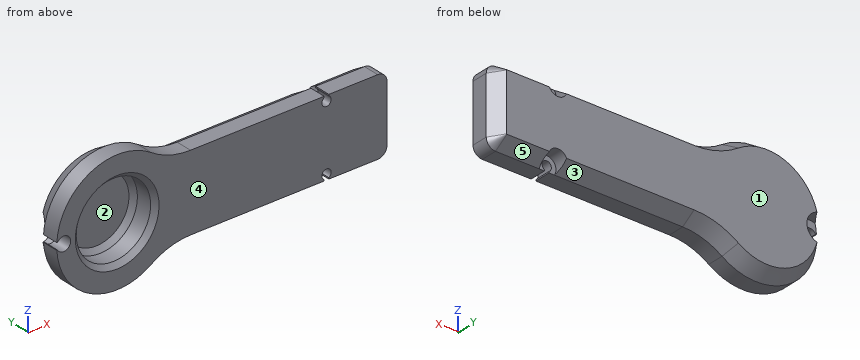
from build123d import *
from OCP.BRepFilletAPI import BRepFilletAPI_MakeChamfer

# Parameters (mm, degrees)
BOSS_EXTRUDE1_DEPTH = 6.5
SKETCH3_R           = 8
CUT_EXTRUDE2_DEPTH  = 5.5
CHAMFER4_SIZE       = 1
FILLET3_R           = 2
FILLET4_R           = 15
CHAMFER7_SIZE       = 3
CHAMFER7_SIZE2      = 1.94822278
SKETCH4_R           = 2
SKETCH4_R_2         = 3
CUT_EXTRUDE7_DEPTH  = 3


with BuildPart() as part:
    # Sketch1 → Boss-Extrude1 (new body)
    with BuildSketch(Plane(origin=(0, 0, 0), x_dir=(1, 0, 0), z_dir=(0, 1, 0))):
        with BuildLine():
            Line((10.132076539, 8.145), (44.5, 8.145))
            Line((44.5, 8.145), (44.5, 7.866025404))
            ThreePointArc((44.5, 7.866025404), (45, 6), (45.5, 7.866025404))
            Line((45.5, 7.866025404), (45.5, 8.145))
            Line((45.5, 8.145), (58, 8.145))
            Line((58, 8.145), (58, -8.145))
            Line((58, -8.145), (45.5, -8.145))
            Line((45.5, -8.145), (45.5, -7.866025404))
            ThreePointArc((45.5, -7.866025404), (45, -6), (44.5, -7.866025404))
            Line((44.5, -7.866025404), (44.5, -8.145))
            Line((44.5, -8.145), (10.132076539, -8.145))
            ThreePointArc((10.132076539, -8.145), (-3.961921331, -12.381566111), (-12.978347352, -0.75))
            Line((-12.978347352, -0.75), (-12.799038106, -0.75))
            ThreePointArc((-12.799038106, -0.75), (-10, 0), (-12.799038106, 0.75))
            Line((-12.799038106, 0.75), (-12.978347352, 0.75))
            ThreePointArc((-12.978347352, 0.75), (-3.961921331, 12.381566111), (10.132076539, 8.145))
        make_face()
    extrude(amount=BOSS_EXTRUDE1_DEPTH)

    # Sketch3 → Cut-Extrude2 (cut)
    with BuildSketch(Plane.XZ):
        with Locations(Location((0, 0, 0), (0, 0, 270))):
            Circle(SKETCH3_R)
    extrude(amount=-CUT_EXTRUDE2_DEPTH, mode=Mode.SUBTRACT)

    # Chamfer4
    chamfer4_edges = [part.edges().sort_by_distance(p)[0] for p in [
        (0, 5.5, 8),
        (0, 0, 8),
    ]]
    chamfer(chamfer4_edges, length=CHAMFER4_SIZE)

    # Fillet3
    fillet3_edges = [part.edges().sort_by_distance(p)[0] for p in [
        (58, 3.25, -8.145),
        (58, 3.25, 8.145),
    ]]
    fillet(fillet3_edges, radius=FILLET3_R)

    # Fillet4
    fillet4_edges = [part.edges().sort_by_distance(p)[0] for p in [
        (10.132076539, 3.25, -8.145),
        (10.132076539, 3.25, 8.145),
    ]]
    fillet(fillet4_edges, radius=FILLET4_R)

    # Chamfer7: one chamfer whose edges measure the first distance from different faces: ONE call of the kernel's chamfer builder (chamfer() names one face for all edges)
    chamfer7_edges_1 = [part.edges().sort_by_distance(p)[0] for p in [
        (-5.74409604, 6.5, -11.662133625),
    ]]
    chamfer7_side_1 = [part.faces().sort_by_distance(p)[0] for p in [
        (-5.74409604, 3.25, -11.662133625),
    ]]
    chamfer7_edges_2 = [part.edges().sort_by_distance(p)[0] for p in [
        (11.341184071, 6.5, -8.80996238),
    ]]
    chamfer7_side_2 = [part.faces().sort_by_distance(p)[0] for p in [
        (11.341184071, 3.25, -8.80996238),
    ]]
    chamfer7_edges_3 = [part.edges().sort_by_distance(p)[0] for p in [
        (30.12891133, 6.5, -8.145),
    ]]
    chamfer7_side_3 = [part.faces().sort_by_distance(p)[0] for p in [
        (30.12891133, 3.25, -8.145),
    ]]
    chamfer7_edges_4 = [part.edges().sort_by_distance(p)[0] for p in [
        (50.75, 6.5, -8.145),
    ]]
    chamfer7_side_4 = [part.faces().sort_by_distance(p)[0] for p in [
        (50.75, 3.25, -8.145),
    ]]
    chamfer7_edges_5 = [part.edges().sort_by_distance(p)[0] for p in [
        (57.414213562, 6.5, -7.559213562),
    ]]
    chamfer7_side_5 = [part.faces().sort_by_distance(p)[0] for p in [
        (57.414213562, 3.25, -7.559213562),
    ]]
    chamfer7_edges_6 = [part.edges().sort_by_distance(p)[0] for p in [
        (58, 6.5, 0),
    ]]
    chamfer7_side_6 = [part.faces().sort_by_distance(p)[0] for p in [
        (58, 3.25, 0),
    ]]
    chamfer7_edges_7 = [part.edges().sort_by_distance(p)[0] for p in [
        (57.414213562, 6.5, 7.559213562),
    ]]
    chamfer7_side_7 = [part.faces().sort_by_distance(p)[0] for p in [
        (57.414213562, 3.25, 7.559213562),
    ]]
    chamfer7_edges_8 = [part.edges().sort_by_distance(p)[0] for p in [
        (50.75, 6.5, 8.145),
    ]]
    chamfer7_side_8 = [part.faces().sort_by_distance(p)[0] for p in [
        (50.75, 3.25, 8.145),
    ]]
    chamfer7_edges_9 = [part.edges().sort_by_distance(p)[0] for p in [
        (30.12891133, 6.5, 8.145),
    ]]
    chamfer7_side_9 = [part.faces().sort_by_distance(p)[0] for p in [
        (30.12891133, 3.25, 8.145),
    ]]
    chamfer7_edges_10 = [part.edges().sort_by_distance(p)[0] for p in [
        (11.341184071, 6.5, 8.80996238),
    ]]
    chamfer7_side_10 = [part.faces().sort_by_distance(p)[0] for p in [
        (11.341184071, 3.25, 8.80996238),
    ]]
    chamfer7_edges_11 = [part.edges().sort_by_distance(p)[0] for p in [
        (-5.74409604, 6.5, 11.662133625),
    ]]
    chamfer7_side_11 = [part.faces().sort_by_distance(p)[0] for p in [
        (-5.74409604, 3.25, 11.662133625),
    ]]
    chamfer7 = BRepFilletAPI_MakeChamfer(part.part.solid().wrapped)
    for e in chamfer7_edges_1:
        chamfer7.Add(CHAMFER7_SIZE, CHAMFER7_SIZE2, e.wrapped, chamfer7_side_1[0].wrapped)  # the first distance lies on this face
    for e in chamfer7_edges_2:
        chamfer7.Add(CHAMFER7_SIZE, CHAMFER7_SIZE2, e.wrapped, chamfer7_side_2[0].wrapped)  # the first distance lies on this face
    for e in chamfer7_edges_3:
        chamfer7.Add(CHAMFER7_SIZE, CHAMFER7_SIZE2, e.wrapped, chamfer7_side_3[0].wrapped)  # the first distance lies on this face
    for e in chamfer7_edges_4:
        chamfer7.Add(CHAMFER7_SIZE, CHAMFER7_SIZE2, e.wrapped, chamfer7_side_4[0].wrapped)  # the first distance lies on this face
    for e in chamfer7_edges_5:
        chamfer7.Add(CHAMFER7_SIZE, CHAMFER7_SIZE2, e.wrapped, chamfer7_side_5[0].wrapped)  # the first distance lies on this face
    for e in chamfer7_edges_6:
        chamfer7.Add(CHAMFER7_SIZE, CHAMFER7_SIZE2, e.wrapped, chamfer7_side_6[0].wrapped)  # the first distance lies on this face
    for e in chamfer7_edges_7:
        chamfer7.Add(CHAMFER7_SIZE, CHAMFER7_SIZE2, e.wrapped, chamfer7_side_7[0].wrapped)  # the first distance lies on this face
    for e in chamfer7_edges_8:
        chamfer7.Add(CHAMFER7_SIZE, CHAMFER7_SIZE2, e.wrapped, chamfer7_side_8[0].wrapped)  # the first distance lies on this face
    for e in chamfer7_edges_9:
        chamfer7.Add(CHAMFER7_SIZE, CHAMFER7_SIZE2, e.wrapped, chamfer7_side_9[0].wrapped)  # the first distance lies on this face
    for e in chamfer7_edges_10:
        chamfer7.Add(CHAMFER7_SIZE, CHAMFER7_SIZE2, e.wrapped, chamfer7_side_10[0].wrapped)  # the first distance lies on this face
    for e in chamfer7_edges_11:
        chamfer7.Add(CHAMFER7_SIZE, CHAMFER7_SIZE2, e.wrapped, chamfer7_side_11[0].wrapped)  # the first distance lies on this face
    add(Compound.cast(chamfer7.Shape()), mode=Mode.REPLACE)

    # Sketch4 → Cut-Extrude7 (cut)
    with BuildSketch(Plane(origin=(0, 6.5, 0), x_dir=(1, 0, 0), z_dir=(0, 1, 0))):
        with Locations((45, 7)):
            Circle(SKETCH4_R)
        with Locations((45, -7)):
            Circle(SKETCH4_R)
        with Locations((-11.5, 0)):
            Circle(SKETCH4_R_2)
    extrude(amount=-CUT_EXTRUDE7_DEPTH, mode=Mode.SUBTRACT)


solid = part.part
Work out the finished part from the listing and answer in its coordinate system (mm). Face numbers are marked on the shaded views. A direction names the side the tool comes from. Round coordinates to 2 decimals unless told otherwise and drop trailing zeros. Write each loop counter-clockwise with the first axis right and the second up, starting at its lowest first coordinate (ties: lowest second). Pieces come first, ordered by that corner, then holes. Notation, with made-up numbers: (28, -11.75) -> (87, -11.75) arc R29 ccw to (87, 14.25) -> close; hole circle Ø11 at (31.5, -5). An arc over 180 degrees is marked (long way). Write each question's results on one line, items separated by ' | '.
Item 1: A cutting plane is placed at C-C, the plane x = 37. Determine the outline of the cut face in (y, z) (3 decimals).
Result set:
outline: (0, -8.145) -> (3.5, -8.145) -> (6.5, -6.197) -> (6.5, 6.197) -> (3.5, 8.145) -> (0, 8.145) -> close
Item 2: Flat-ended cylindrical pins translate along their axes: P1, Ø1.8, axis at x = 52.5, y = 1.5, coming from the -Z side (3 decimals); P2, Ø5, axis at x = -11.5, z = 0, coming from the +Y side; P3, Ø1, axis at x = 30, y = 5.5, coming from the -Z side. Find the tip coordinate at first contact, or state that the pin passes through.
Result set:
P1: z = -8.145 | P2: y = 3.5 | P3: z = -7.17
Item 3: Find the intervals of material crossed by line 1 along X through (y, z) = (3.25, -4.25); line 2 along Z through (x, y) = (-11.5, 2.5); line 3 along Z through (x, y) = (27.5, 2.5) (3 decimals), in increasing order. Write a range as [from, to].
Result set:
line 1: [-12.29, -6.78], [6.78, 58] | line 2: [-6.06, -1.5], [1.5, 6.06] | line 3: [-8.145, 8.145]
Item 4: A cutting plane is placed at A-A, the plane z = 0. Determine the outline of the cut face in (x, y).
Result set:
outline: (-10, 0) -> (-9, 0) -> (-8, 1) -> (-8, 4.5) -> (-7, 5.5) -> (7, 5.5) -> (8, 4.5) -> (8, 1) -> (9, 0) -> (58, 0) -> (58, 3.5) -> (56.05, 6.5) -> (-8.5, 6.5) -> (-8.5, 3.5) -> (-10, 3.5) -> close
Item 5: Which of the six approach directions +Z, -Z, +X, -X, +Y, -Y give full straight-line access (tool end or side, diameter ignored) to the marked faces 4 and 5?
Result set:
face 4: +Z, -Z, +X, -X, -Y | face 5: -Z, +X, +Y
Item 6: A cutting plane is placed at B-B, the plane x = 0. Determine the outline of the cut face in (y, z), plus the area to 3 significant figures.
Result set:
outline: (0, -13) -> (3.5, -13) -> (6.5, -11.05) -> (6.5, 11.05) -> (3.5, 13) -> (0, 13) -> (0, 9) -> (1, 8) -> (4.5, 8) -> (5.5, 7) -> (5.5, -7) -> (4.5, -8) -> (1, -8) -> (0, -9) -> close | area: 75.2 mm^2
Item 7: The mould has two halves that part along Z. Classify the marked faces 1, 2 and 3: +Z half, -Z half, draft (parallel to the pull), parting line (faces both ways), or undercut.
Result set:
face 1: draft | face 2: undercut | face 3: -Z half
